from build123d import *

# Parameters (mm, degrees)
SKETCH1_W           = 72
SKETCH1_H           = 4
BOSS_EXTRUDE1_DEPTH = 12
SKETCH2_W           = 10.7
SKETCH2_H           = 44.65
BOSS_EXTRUDE2_DEPTH = 5


with BuildPart() as part:
    # Sketch1 → Boss-Extrude1 (new body, symmetric)
    with BuildSketch(Plane(origin=(0, 0, 0), x_dir=(0, 0, -1), z_dir=(1, 0, 0))):
        with Locations((36, 2)):
            Rectangle(SKETCH1_W, SKETCH1_H)
    extrude(amount=BOSS_EXTRUDE1_DEPTH, both=True)

    # Sketch2 → Boss-Extrude2 (add)
    with BuildSketch(Plane(origin=(0, 0, 0), x_dir=(1, 0, 0), z_dir=(0, 1, 0))):
        with BuildLine():
            ThreePointArc((-5.35, 44.65), (0, 50), (5.35, 44.65))
            Line((5.35, 44.65), (-5.35, 44.65))
        make_face()
        with Locations((0, 22.325)):
            Rectangle(SKETCH2_W, SKETCH2_H)
    extrude(amount=-BOSS_EXTRUDE2_DEPTH)


solid = part.part
The listing builds one solid part. Answer for the finished solid, in the listing's coordinates (mm). A direction names the side the tool comes from. Give positions to 0.01 mm unless a question says otherwise; leave off trailing zeros. Write each loop counter-clockwise with the first axis right and the second up, starting at its lowest first coordinate (ties: lowest second). Pieces come first, ordered by that corner, then holes.
Item 1: Section A-A, the plane x = 0 is taken. Write down the section's boundary in (y, z), plus the area to 3 significant figures.
Item 2: Section C-C, the plane y = -4 is taken. Write down the section's boundary in (x, z).
Item 3: Section B-B, the plane z = -43 is taken. Write down the section's boundary in (x, y).
Item 4: Which of the six approach directions +Z, -Z, +X, -X, +Y, -Y give full straight-line access (tool end or side, diameter ignored) to faces 1 (the flat face through (5.35, -2, -22)), 2 (the flat face through (-5.35, -2, -22)), 3 (the cylindrical face through (0, -2, -50))?
Item 5: Find the intervals of material crossed by line 1 along Z through (x, y) = (-0.25, -1); line 2 along Y through (x, z) = (10.25, -55.5); line 3 along X through (y, z) = (-4, -43.5), in increasing order.
Item 6: Flat-ended cylindrical pins translate along their axes: P1, Ø1.5, axis at x = 5, y = -3, coming from the -Z side; P2, Ø4, axis at y = -2.5, z = -24.5, coming from the +X side; P3, Ø1.5, axis at y = -1.5, z = -16.5, coming from the -X side. Find the tip coordinate at first contact, or state that the pin passes through.
Item 7: Section D-D, the plane z = -66 is taken. Write down the section's boundary in (x, y).
Completed:
1. outline: (-5, -50) - (0, -50) - (0, -72) - (4, -72) - (4, 0) - (-5, 0) - close
1. area: 538 mm2
2. outline: (-5.35, -44.65) arc R5.35 ccw to (5.35, -44.65) - (5.35, 0) - (-5.35, 0) - close
3. outline: (-12, 0) - (-5.35, 0) - (-5.35, -5) - (5.35, -5) - (5.35, 0) - (12, 0) - (12, 4) - (-12, 4) - close
4. face 1: +Z, -Z, +X, -Y
4. face 2: +Z, -Z, -X, -Y
4. face 3: -Z, -Y
5. line 1: z = -49.99 to 0
5. line 2: y = 0 to 4
5. line 3: x = -5.35 to 5.35
6. P1: stops at z = -47.9
6. P2: stops at x = 5.35
6. P3: stops at x = -5.35
7. outline: (-12, 0) - (12, 0) - (12, 4) - (-12, 4) - close
